Could you check a few things on this model? Use its own coordinates, in mm. A direction names the side the tool comes from. Round coordinates to 2 decimals unless told otherwise and drop trailing zeros. Write each loop counter-clockwise with the first axis right and the second up, starting at its lowest first coordinate (ties: lowest second). Pieces come first, ordered by that corner, then holes. Notation, with made-up numbers: (88.5, 41.25) - (129.5, 41.25) arc R4 cw to (129.5, 45.25) - close; hole circle Ø7 at (-10.75, -21.75). An arc over 180 degrees is marked (long way). Put each result on its own line as item: value.
from build123d import *

# Parameters (mm, degrees)
SKETCH_1_R          = 1.5
EXTRUDE_1_DEPTH     = 3.8
EXTRUDE_2_DEPTH     = 8
SKETCH_3_R          = 3.25
CUT_EXTRUDE_1_DEPTH = 49.22207155
SKETCH_4_R          = 4.25
CUT_EXTRUDE_2_DEPTH = 2
FILLET_2_R          = 1
FILLET_3_R          = 2
FILLET_4_R          = 5
FILLET_5_R          = 2
SKETCH_5_R          = 2.5
SKETCH_5_R_2        = 1.5
CUT_EXTRUDE_3_DEPTH = 52.897670319


with BuildPart() as part:
    # 草图1 → 凸台-拉伸1 (new body)
    with BuildSketch(Plane.XY):
        with BuildLine():
            Line((35.721518987, -3), (42.721518987, -3))
            Line((42.721518987, -3), (42.721518987, 0))
            Line((42.721518987, 0), (35.721518987, 0))
            Line((35.721518987, 0), (35.721518987, 8))
            Line((35.721518987, 8), (-9.278481013, 8))
            Line((-9.278481013, 8), (-9.278481013, -3))
            Line((-9.278481013, -3), (-9.278481013, -12.5))
            ThreePointArc((-9.278481013, -12.5), (-2.778481013, -19), (3.721518987, -12.5))
            Line((3.721518987, -12.5), (3.721518987, -3))
            Line((3.721518987, -3), (35.721518987, -3))
        make_face()
        with Locations(Location((0.221518987, -13, 0), (0, 0, 180))):
            Circle(SKETCH_1_R, mode=Mode.SUBTRACT)
    extrude(amount=EXTRUDE_1_DEPTH)

    # 草图2 → 凸台-拉伸2 (add)
    with BuildSketch(Plane.XY.offset(3.8)):
        Polygon((3.721518987, -3), (-9.278481013, -3), (-9.278481013, 8), (35.721518987, 8), (35.721518987, 0), (42.721518987, 0), (42.721518987, -3), align=None)
    extrude(amount=EXTRUDE_2_DEPTH)

    # 草图3 → 切除-拉伸1 (cut, through all)
    with BuildSketch(Plane.XY.offset(11.8)):
        with Locations((-4.278481013, 3)):
            Circle(SKETCH_3_R)
    extrude(amount=-CUT_EXTRUDE_1_DEPTH, mode=Mode.SUBTRACT)

    # 草图4 → 切除-拉伸2 (cut)
    with BuildSketch(Plane.XY.offset(11.8)):
        with Locations((-4.278481013, 3)):
            Circle(SKETCH_4_R)
    extrude(amount=-CUT_EXTRUDE_2_DEPTH, mode=Mode.SUBTRACT)

    # 圆角2
    fillet_2_edges = [part.edges().sort_by_distance(p)[0] for p in [
        (-9.278481013, 8, 5.9),
        (-9.278481013, -3, 7.8),
    ]]
    fillet(fillet_2_edges, radius=FILLET_2_R)

    # 圆角3
    fillet_3_edges = [part.edges().sort_by_distance(p)[0] for p in [
        (35.721518987, 8, 5.9),
    ]]
    fillet(fillet_3_edges, radius=FILLET_3_R)

    # 圆角4
    fillet_4_edges = [part.edges().sort_by_distance(p)[0] for p in [
        (35.721518987, 0, 5.9),
    ]]
    fillet(fillet_4_edges, radius=FILLET_4_R)

    # 圆角5
    fillet_5_edges = [part.edges().sort_by_distance(p)[0] for p in [
        (42.721518987, 0, 5.9),
    ]]
    fillet(fillet_5_edges, radius=FILLET_5_R - 0.0001)  # a hair under: the kernel refuses the full size

    # 草图5 → 切除-拉伸3 (cut, through all)
    with BuildSketch(Plane(origin=(0, 8, 0), x_dir=(1, 0, 0), z_dir=(0, 1, 0))):
        with Locations(Location((5.721518987, -5.9, 0), (0, 0, 180))):
            Circle(SKETCH_5_R)
        with Locations(Location((21.721518987, -5.9, 0), (0, 0, 180))):
            Circle(SKETCH_5_R_2)
    extrude(amount=-CUT_EXTRUDE_3_DEPTH, mode=Mode.SUBTRACT)


solid = part.part
(1) For faces 5 (the face through (35.722, 5.5, 5.8)), 6 (the face through (3.722, -8, 2)), 7 (the face through (-0.225, 4.277, 10.814)), which set-ups out of +Z, -Z, +X, -X, +Y, -Y let a thin tool reach every point of the face, with its end or its side?
Values found:
face 5: +Z, -Z, +X, +Y
face 6: +Z, -Z, +X, -Y
face 7: +Z
(2) I'm going to push flat-ended pins straight in: pin 1 (2 mm diameter, centred on x = 24.5, z = 6, fed in from -Y); pin 2 (10.5 mm diameter, centred on x = -4.5, y = -11.5, fed in from +Z); pin 3 (0.5 mm diameter, centred on y = 5.5, z = 7.5, fed in from +X). Where does each tip first touch, or does it pass through?
Values found:
pin 1: stops at y = -3
pin 2: stops at z = 3.8
pin 3: stops at x = 35.72
(3) Imagine slicing it at A-A, the plane z = 5.9. Give the number of separate pieces and of enclosed holes in the cut face, then the cut area to 3 significant figures.
Values found:
separate pieces: 3
enclosed holes: 1
area: 398 mm^2
(4) If we mould it in two halves opening along Z, with no side actions, what happens to faces 1 (the face through (6.26, 2.58, 3.46)), 2 (the face through (-2.9, -19, 1.9)), 3 (the face through (-3, -10, 3.8)), 4 (the face through (23.22, 2.58, 5.97))? For each: pulls with the +Z half, pulls with the -Z half, needs draft (parallel to the pull), parting line crosses it, or undercut.
Values found:
face 1: undercut
face 2: needs draft
face 3: pulls with the +Z half
face 4: undercut
(5) Imagine slicing it at B-B, the plane y = 4.25. List the corners of the cut face in (x, z) for me.
Values found:
outline: (-9.28, 0) - (-7.28, 0) - (-7.28, 9.8) - (-8.34, 9.8) - (-8.34, 11.8) - (-9.28, 11.8) - close; (-1.28, 0) - (35.78, 0) - (35.78, 11.8) - (-0.22, 11.8) - (-0.22, 9.8) - (-1.28, 9.8) - close; hole circle Ø5 at (5.72, 5.9); hole circle Ø3 at (21.72, 5.9)
(6) Please list where these lines run through material, in increasing order: probe 1 along X at (y, z) = (0.5, 4); probe 2 along Y at (x, z) = (13.5, 8.5); probe 3 along Z at (x, y) = (21.5, 2.5). Write a range as from..to.
Values found:
probe 1: x = -9.28..-6.36, -2.2..4.1, 7.35..38.54
probe 2: y = -3..8
probe 3: z = 0..4.42, 7.38..11.8
(7) Imagine slicing it at D-D, the plane y = -13. List the corners of the cut face in (x, z) for me, then the cut area to 3 significant figures.
Values found:
outline: (-9.26, 0) - (-1.28, 0) - (-1.28, 3.8) - (-9.26, 3.8) - close; (1.72, 0) - (3.7, 0) - (3.7, 3.8) - (1.72, 3.8) - close
area: 37.9 mm^2
